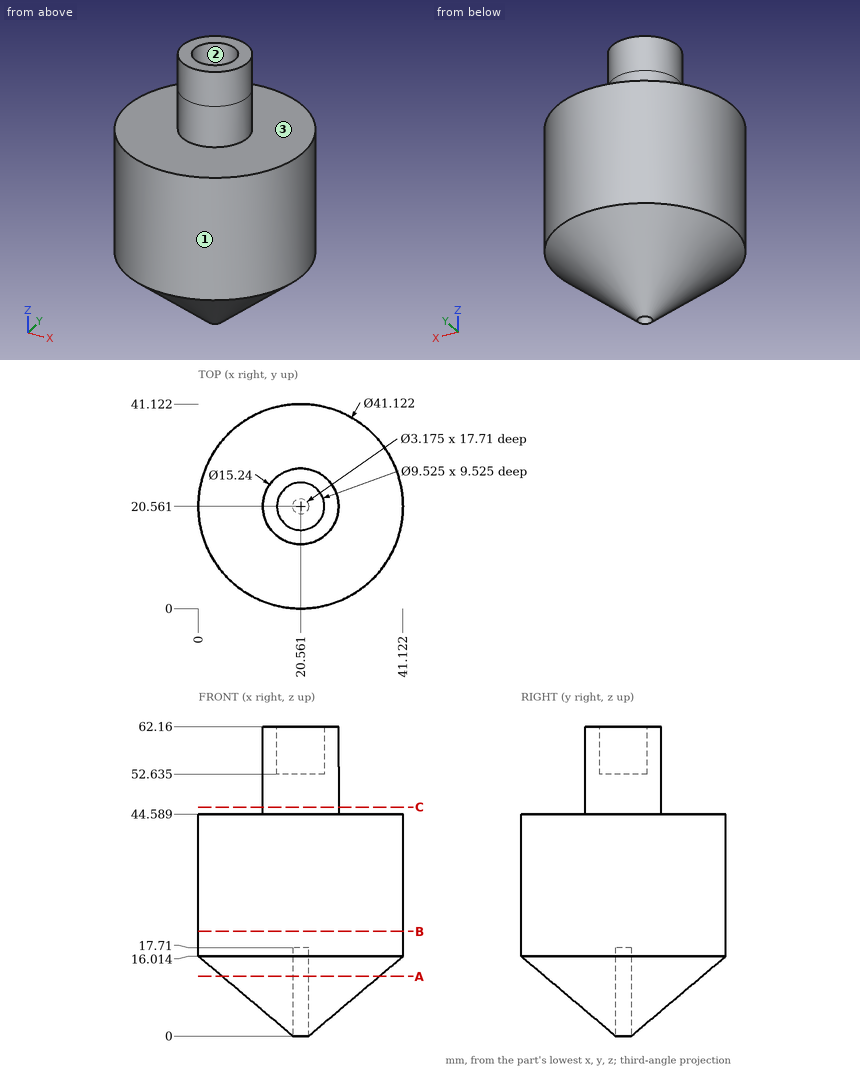
Could you check a few things on this drawing? It's one solid part, dimensions in mm from its lowest x, y, z. Round coordinates to 2 decimals unless told otherwise and drop trailing zeros. Loops run counter-clockwise (first coordinate to the right, second up) from the corner with the lowest first, then second, coordinate; pieces in that order, holes last. Notation, with made-up numbers: M 14,54 L 46,54 A9 cw 46,66 Z; hole C 64,65.5 d1. An arc over 180 degrees is marked long. Write each question's results on one line, items separated by ' | '. Start each with the question number.
(1) I want a section at A-A (z = 12). Please give me the cut outline in (x, y) (1 decimal).
(2) If I drill on probe 1 along Y at (x, z) = (21.5, 11.5) (1 decimal); probe 2 along X at (y, z) = (27, 38.5) (1 decimal); probe 3 along Y at (x, z) = (32.5, 11) (1 decimal), over which ranges is the centre line in solid material (lowest first)? Write a range as from..to.
(3) Will these pins go through, and if not, where does the flat tip stop? P1, Ø2, axis at x = 15, z = 9.5, coming from the +Y side (1 decimal); P2, Ø5, axis at y = 25, z = 24.5, coming from the +X side; P3, Ø12, axis at x = 25, z = 11, coming from the +Y side.
(4) I want a section at C-C (z = 46). Please give me the cut outline in (x, y).
(5) I want a section at B-B (z = 21). Please give me the cut outline in (x, y), then the cut area to 3 significant figures.
(6) Thinking about a two-plate mould opening in X: for the marked faces 1, 2 and 3, which applies, pulls with the +X half, pulls with the -X half, needs draft (parallel to the pull), parting line crosses it, or undercut?
Solved:
1) outline: C 20.6,20.6 d31.6; hole C 20.6,20.6 d3.2
2) probe 1: y = 5.4..19.3, 21.8..35.7 | probe 2: x = 1..40.1 | probe 3: y = 12.1..29
3) P1: stops at y = 33.5 | P2: stops at x = 41.03 | P3: stops at y = 41.09
4) outline: C 20.56,20.56 d15.24
5) outline: C 20.56,20.56 d41.12 | area: 1,330 mm²
6) face 1: parting line crosses it | face 2: undercut | face 3: needs draft
